Source: CAD feature listing. Evaluate the final solid. Frame: model axes, mm. Face numbers are marked on the shaded views. A direction names the side the tool comes from. Give positions to 0.01 mm unless a question says otherwise; leave off trailing zeros. Order: outer loops, then holes, each group sorted by start corner. A loop starts at its lowest first (then second) coordinate and runs counter-clockwise, first axis right, second up. Notation, with made-up numbers: M 29,50.25 L 73,50.25 A22 ccw 73,89.25 Z; hole C -32.75,-15.75 d4. An arc over 180 degrees is marked long. Return JSON: item names as keys, results as strings.
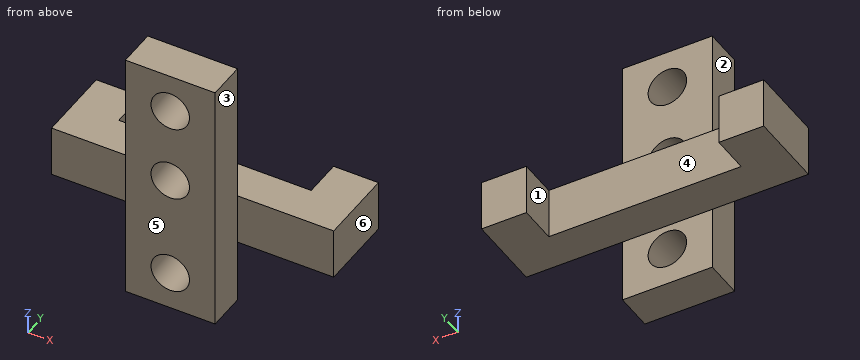
from build123d import *

# Parameters (mm, degrees)
SKETCH2_W                    = 7
SKETCH2_H                    = 20
EXTRUDE2_DEPTH               = 3
F_3_0_3_DIAMETER_HOLE1_D     = 3
F_3_0_3_DIAMETER_HOLE1_DEPTH = 10
F_3_0_3_DIAMETER_HOLE1_TIP   = 0.901290929
SKETCH6_W                    = 7
SKETCH6_H                    = 4
EXTRUDE3_DEPTH               = 6
SKETCH7_W                    = 4
SKETCH7_H                    = 6
EXTRUDE4_DEPTH               = 7.5
SKETCH8_W                    = 4
SKETCH8_H                    = 6
EXTRUDE5_DEPTH               = 7.5
SKETCH10_W                   = 15
SKETCH10_H                   = 4
EXTRUDE6_DEPTH               = 3


with BuildPart() as part:
    # Sketch2 → Extrude2 (new body)
    with BuildSketch(Plane(origin=(0, 0, 0), x_dir=(1, 0, 0), z_dir=(0, 1, 0))):
        Rectangle(SKETCH2_W, SKETCH2_H)
    extrude(amount=EXTRUDE2_DEPTH)

    # Ø3.0 (3) Diameter Hole1
    with Locations(Plane(origin=(0, 3, 7), x_dir=(0, 0, 1), z_dir=(0, 1, 0))):
        with Locations((0, 0), (-6, 0), (-14, 0)):
            Hole(F_3_0_3_DIAMETER_HOLE1_D / 2, depth=F_3_0_3_DIAMETER_HOLE1_DEPTH)
            with Locations((0, 0, -(F_3_0_3_DIAMETER_HOLE1_DEPTH + F_3_0_3_DIAMETER_HOLE1_TIP / 2))):  # 118° drill point
                Cone(0, F_3_0_3_DIAMETER_HOLE1_D / 2, F_3_0_3_DIAMETER_HOLE1_TIP, mode=Mode.SUBTRACT)

    # Sketch6 → Extrude3 (add)
    with BuildSketch(Plane(origin=(0, 3, 0), x_dir=(1, 0, 0), z_dir=(0, 1, 0))):
        with Locations((0, 3)):
            Rectangle(SKETCH6_W, SKETCH6_H)
    extrude(amount=EXTRUDE3_DEPTH)

    # Sketch7 → Extrude4 (add)
    with BuildSketch(Plane(origin=(3.5, 0, 0), x_dir=(0, 0, -1), z_dir=(1, 0, 0))):
        with Locations((3, 6)):
            Rectangle(SKETCH7_W, SKETCH7_H)
    extrude(amount=EXTRUDE4_DEPTH)

    # Sketch8 → Extrude5 (add)
    with BuildSketch(Plane.ZY.offset(3.5)):
        with Locations((-3, 6)):
            Rectangle(SKETCH8_W, SKETCH8_H)
    extrude(amount=EXTRUDE5_DEPTH)

    # Sketch10 → Extrude6 (cut)
    with BuildSketch(Plane(origin=(0, 9, 0), x_dir=(-1, 0, 0), z_dir=(0, 1, 0))):
        with Locations((0, -3)):
            Rectangle(SKETCH10_W, SKETCH10_H)
    extrude(amount=-EXTRUDE6_DEPTH, mode=Mode.SUBTRACT)


solid = part.part
1. Set-up query: the marked faces 1, 2 and 3. Return all of +Z, -Z, +X, -X, +Y, -Y with unobstructed straight access to the full face (end or side cutting, diameter ignored); none if empty.
Evaluation:
{"face 1": "+Z, -Z, +Y", "face 2": "+Z, -Z, -X, -Y", "face 3": "+Z, -Z, +X, -Y"}
2. Draft query along X for the marked faces 4, 5 and 6. Return one class per face: pulls with the +X half, pulls with the -X half, needs draft (parallel to the pull), parting line crosses it, or undercut.
Evaluation:
{"face 4": "undercut", "face 5": "needs draft", "face 6": "pulls with the +X half"}
3. Section query A-A (x = 0). Return loops of the section in (y, z), then the cut area to 3 significant figures.
Evaluation:
{"outline": "M 0,-10 L 3,-10 L 3,-8.5 L 0,-8.5 Z; M 0,-5.5 L 3,-5.5 L 3,-5 L 6,-5 L 6,-1 L 3,-1 L 3,-0.5 L 0,-0.5 Z; M 0,2.5 L 3,2.5 L 3,5.5 L 0,5.5 Z; M 0,8.5 L 3,8.5 L 3,10 L 0,10 Z", "area": "45.0 mm^2"}
4. First-contact query: pin 1 (1.2 mm diameter, centred on x = 1.5, z = -3, fed in from +Y); pin 2 (5 mm diameter, centred on x = 2.5, z = 5.5, fed in from +Y); pin 3 (1.8 mm diameter, centred on x = 0, z = -7, fed in from +Y); pin 4 (1.2 mm diameter, centred on x = 8.5, z = -2.5, fed in from -Y). Flat tips, straight axial feed; report the tip coordinate or a pass-through.
Evaluation:
{"pin 1": "stops at y = 6", "pin 2": "stops at y = 3", "pin 3": "passes through", "pin 4": "stops at y = 3"}
5. Ray query, probe 1 along X at (y, z) = (1.2, -7); probe 2 along X at (y, z) = (1.5, 3.25); probe 3 along Y at (x, z) = (-3.25, -1.5). Return the intervals inside material, ascending.
Evaluation:
{"probe 1": "x = -3.5 to -1.5, 1.5 to 3.5", "probe 2": "x = -3.5 to 3.5", "probe 3": "y = 0 to 6"}
6. Section query D-D (y = 7). Return loops of the section in (x, z).
Evaluation:
{"outline": "M -11,-5 L -7.5,-5 L -7.5,-1 L -11,-1 Z; M 7.5,-5 L 11,-5 L 11,-1 L 7.5,-1 Z"}
7. Section query C-C (z = -7). Return loops of the section in (x, y), then the cut area to 3 significant figures.
Evaluation:
{"outline": "M -3.5,0 L -1.5,0 L -1.5,3 L -3.5,3 Z; M 1.5,0 L 3.5,0 L 3.5,3 L 1.5,3 Z", "area": "12.0 mm^2"}
8. Section query B-B (y = 2.75). Return loops of the section in (x, z).
Evaluation:
{"outline": "M -3.5,-10 L 3.5,-10 L 3.5,10 L -3.5,10 Z; hole C 0,-7 d3; hole C 0,1 d3; hole C 0,7 d3"}
